```python
from build123d import *

# Parameters (mm, degrees)
SKETCH_1_R                     = 12
SKETCH_1_R_2                   = 3
EXTRUDE_1_DEPTH                = 4.2
SKETCH_2_R                     = 5
EXTRUDE_2_DEPTH                = 2
HOLE_WIZARD_M2_5_1_D           = 2.7
HOLE_WIZARD_M2_5_1_CBORE_D     = 5
HOLE_WIZARD_M2_5_1_CBORE_DEPTH = 2.5
PATTERN_CIRCULAR_1_COUNT       = 4
CHAMFER_3_SIZE                 = 0.2
SKETCH_12_R                    = 2.5
EXTRUDE_1662_DEPTH             = 26
CUT_EXTRUDE_START              = -15
CUT_EXTRUDE_1_DEPTH            = 15


with BuildPart() as part:
    # 草图1 → 凸台-拉伸1 (new body)
    # profile 1 of 2: a face of its own
    with BuildSketch(Plane.XY):
        Circle(SKETCH_1_R)
        Circle(SKETCH_1_R_2, mode=Mode.SUBTRACT)
    # profile 2 of 2: a face of its own
    with BuildSketch(Plane.XY):
        Circle(SKETCH_1_R_2)
    extrude(amount=EXTRUDE_1_DEPTH)

    # 草图2 → 凸台-拉伸2 (add)
    with BuildSketch(Plane.XY.offset(4.2)):
        Circle(SKETCH_2_R)
    extrude(amount=EXTRUDE_2_DEPTH)

    # M2.5 六角圆柱头螺钉的柱形沉头孔1 (through all)
    with Locations(Plane.XY.offset(4.2)):
        with Locations((0, 8)):
            hole_wizard_m2_5_1 = CounterBoreHole(HOLE_WIZARD_M2_5_1_D / 2, HOLE_WIZARD_M2_5_1_CBORE_D / 2, HOLE_WIZARD_M2_5_1_CBORE_DEPTH)

    # 阵列(圆周)1: M2.5 六角圆柱头螺钉的柱形沉头孔1 ×4 about axis
    pattern_circular_1_axis = Axis((0, 0, 0), (0, 0, 1))
    for i in range(1, PATTERN_CIRCULAR_1_COUNT):
        add(hole_wizard_m2_5_1.rotate(pattern_circular_1_axis, i * 360 / PATTERN_CIRCULAR_1_COUNT), mode=Mode.SUBTRACT)

    # 倒角3
    chamfer_3_edges = [part.edges().sort_by_distance(p)[0] for p in [
        (-12, 0, 0),
        (-12, 0, 4.2),
    ]]
    chamfer(chamfer_3_edges, length=CHAMFER_3_SIZE)

    # 草图12 → Extrude 1662 (add)
    with BuildSketch(Plane.XY.offset(4.2)):
        with Locations(Location((0, 0, 0), (0, 0, 180))):
            Circle(SKETCH_12_R)
    extrude(amount=EXTRUDE_1662_DEPTH)

    # 草图13 → 切除-拉伸1 (cut)
    with BuildSketch(Plane.XY.offset(30.2).offset(CUT_EXTRUDE_START)):
        with BuildLine():
            Line((1.5, 2), (1.5, -2))
            ThreePointArc((1.5, -2), (2.5, 0), (1.5, 2))
        make_face()
    extrude(amount=CUT_EXTRUDE_1_DEPTH, mode=Mode.SUBTRACT)


solid = part.part
```
For this review, take the finished solid that the model builds, in its own axes (mm). A direction names the side the tool comes from. Round coordinates to 2 decimals unless told otherwise and drop trailing zeros. Write each loop counter-clockwise with the first axis right and the second up, starting at its lowest first coordinate (ties: lowest second). Pieces come first, ordered by that corner, then holes. Notation, with made-up numbers: (44, -9) - (91, -9) arc R38 ccw to (91, 29) - close; hole circle Ø2 at (-3, 11.25). An arc over 180 degrees is marked (long way). Put each result on its own line as item: value.
Q1. Insertion check: pin 1 Ø4 at (x, y) = (-1, -8.5) entering from +Z; pin 2 Ø6 at (x, y) = (-7.5, 1) entering from +Z; pin 3 Ø3.5 at (x, y) = (-8, 0) entering from +Z. Each pin has a flat end and moves straight along its axis. Give the tip position at first contact, or say it passes through.
Solved:
pin 1: stops at z = 4.2
pin 2: stops at z = 6.2
pin 3: stops at z = 1.7
Q2. Machinability: for faces 1 (the face through (5, -2, 4.2)), 2 (the face through (9.339, -0.176, 0.838)), which of the approach directions +Z, -Z, +X, -X, +Y, -Y give a long, thin tool a straight path to every point of the face, cutting with its end or side? Answer none if there is none.
Solved:
face 1: +Z
face 2: +Z, -Z
Q3. We need section D-D (z = 16). Give the boundary of the cut face in (x, y).
Solved:
outline: (1.5, -2) - (1.5, 2) arc R2.5 ccw (long way) to start
Q4. Wall thickness on probe 1 along Y at (x, z) = (0, 3.4); probe 2 along Z at (x, y) = (-8.25, -5.25); probe 3 along Y at (x, z) = (8.25, 3): over which ranges is each line inside the solid? List them lowest first.
Solved:
probe 1: y = -12 to -10.5, -5.5 to 5.5, 10.5 to 12
probe 2: z = 0 to 4.2
probe 3: y = -8.71 to -2.49, 2.49 to 8.71
Q5. We need section A-A (z = 3). Give the boundary of the cut face in (x, y).
Solved:
outline: circle Ø24 at (0, 0); hole circle Ø5 at (-8, 0); hole circle Ø5 at (0, -8); hole circle Ø5 at (0, 8); hole circle Ø5 at (8, 0)
Q6. We need section B-B (x = 0). Count the separate pieces of the cut face and the enclosed holes in it, and give its area (3 significant figures).
Solved:
separate pieces: 3
enclosed holes: 0
area: 207 mm2
Q7. Mouldability with a two-part tool opening along Y and no side actions: class faces 3 (the face through (1.5, 0, 23)), 4 (the face through (-1.08, -4.88, 5.19)), 5 (the face through (1.1, 6.9, 1.7)) as released by +Y, released by -Y, zero draft, split by the parting line, or undercut.
Solved:
face 3: zero draft
face 4: split by the parting line
face 5: undercut
